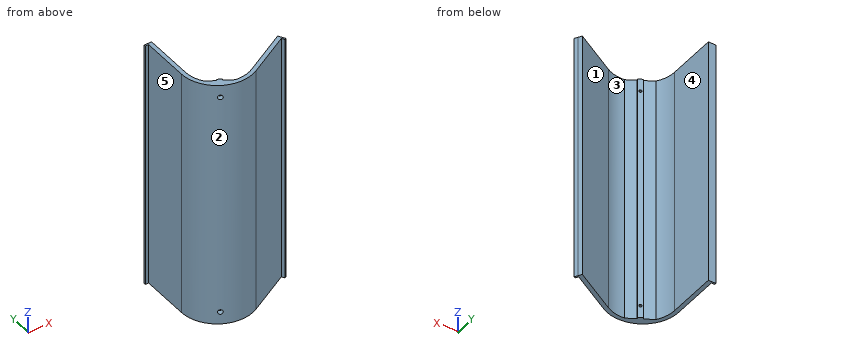
from build123d import *

# Parameters (mm, degrees)
BOSS_EXTRUDE1_DEPTH = 300
SKETCH3_R           = 1.6
CUT_EXTRUDE1_DEPTH  = 27.070508076
CUT_EXTRUDE2_START  = -2
SKETCH4_R           = 2.875
CUT_EXTRUDE2_DEPTH  = 25.070508162
SKETCH5_W           = 6
SKETCH5_H           = 300
SKETCH5_R           = 1.6
BOSS_EXTRUDE2_DEPTH = 2


with BuildPart() as part:
    # Sketch2 → Boss-Extrude1 (new body)
    with BuildSketch(Plane.XY):
        with BuildLine():
            Line((-10, 0), (-10, 57.592991829))
            Line((-10, 57.592991829), (-14, 57.592991829))
            Line((-14, 57.592991829), (-14, 59.592991829))
            Line((-14, 59.592991829), (-10, 59.592991829))
            Line((-10, 59.592991829), (-5, 59.592991829))
            Line((-5, 59.592991829), (-5, 0))
            ThreePointArc((-5, 0), (-3.13691529, -11.76748288), (2.270101024, -22.383928263))
            Line((2.270101024, -22.383928263), (29.120915128, -37.886253013))
            ThreePointArc((29.120915128, -37.886253013), (41.018534684, -37.260643809), (52.141016151, -32.990381057))
            Line((52.141016151, -32.990381057), (103.750060963, -3.193885142))
            Line((103.750060963, -3.193885142), (106.250060963, -7.524012161))
            Line((106.250060963, -7.524012161), (108.250060963, -10.988113776))
            Line((108.250060963, -10.988113776), (106.518010155, -11.988113776))
            Line((106.518010155, -11.988113776), (104.518010155, -8.524012161))
            Line((104.518010155, -8.524012161), (54.641016151, -37.320508076))
            ThreePointArc((54.641016151, -37.320508076), (11.547005384, -37.320508076), (-10, 0))
        make_face()
    extrude(amount=BOSS_EXTRUDE1_DEPTH)

    # Sketch3 → Cut-Extrude1 (cut, through all)
    with BuildSketch(Plane(origin=(-9.125, -15.804963619, 0), x_dir=(0.866025404, -0.5, 0), z_dir=(0.5, 0.866025404, 0))):
        with Locations((28.660254038, -15)):
            Circle(SKETCH3_R)
        with Locations((28.660254038, -285)):
            Circle(SKETCH3_R)
    extrude(amount=-CUT_EXTRUDE1_DEPTH, mode=Mode.SUBTRACT)

    # Sketch4 → Cut-Extrude2 (cut, through all)
    with BuildSketch(Plane(origin=(-9.125, -15.804963619, 0), x_dir=(0.866025404, -0.5, 0), z_dir=(0.5, 0.866025404, 0)).offset(CUT_EXTRUDE2_START)):
        with Locations((28.660254038, -15)):
            Circle(SKETCH4_R)
        with Locations((28.660254038, -285)):
            Circle(SKETCH4_R)
    extrude(amount=-CUT_EXTRUDE2_DEPTH, mode=Mode.SUBTRACT)

    # Sketch5 → Boss-Extrude2 (add)
    with BuildSketch(Plane(origin=(-9.125, -15.804963619, 0), x_dir=(0.866025404, -0.5, 0), z_dir=(0.5, 0.866025404, 0))):
        with Locations((28.660254038, -150)):
            Rectangle(SKETCH5_W, SKETCH5_H)
        with Locations((28.660254038, -15)):
            Circle(SKETCH5_R, mode=Mode.SUBTRACT)
        with Locations((28.660254038, -285)):
            Circle(SKETCH5_R, mode=Mode.SUBTRACT)
    extrude(amount=BOSS_EXTRUDE2_DEPTH)


solid = part.part
Verification items for the finished model (mm, model axes). Face numbers are marked on the shaded views. A direction names the side the tool comes from. Give positions to 0.01 mm unless a question says otherwise; leave off trailing zeros. Loops run counter-clockwise (first coordinate to the right, second up) from the corner with the lowest first, then second, coordinate; pieces in that order, holes last.
1. Material ranges on probe 1 along X at (y, z) = (23, 252.5); probe 2 along X at (y, z) = (-5.5, 170.5); probe 3 along X at (y, z) = (-18.5, 44.5), recorded low to high.
Derived:
probe 1: x = -10 to -5
probe 2: x = -9.65 to -4.6, 99.76 to 105.08
probe 3: x = -5.83 to -0.21, 77.24 to 87.24
2. Tool access check on the marked faces 1 and 2. Record the directions out of +Z, -Z, +X, -X, +Y, -Y that give a thin tool (end or side, any length) a straight path to the whole face; none if there is none.
Derived:
face 1: +Z, -Z, +Y
face 2: +Z, -Z, -Y
3. Cross-section at A-A on z = 61.5. Record the cut outline in (x, y).
Derived:
outline: (-14, 57.59) - (-10, 57.59) - (-10, 0) arc R43.09 ccw to (54.64, -37.32) - (104.52, -8.52) - (106.52, -11.99) - (108.25, -10.99) - (103.75, -3.19) - (52.14, -32.99) arc R38.09 cw to (29.12, -37.89) - (18.29, -31.64) - (19.29, -29.9) - (14.1, -26.9) - (13.1, -28.64) - (2.27, -22.38) arc R38.09 cw to (-5, 0) - (-5, 59.59) - (-14, 59.59) - close
4. Go/stop test with flat-tipped pins: P1, Ø3, axis at x = 50, z = 85.5, coming from the +Y side; P2, Ø8, axis at x = 3, z = 157, coming from the +Y side; P3, Ø12, axis at x = 24, z = 232.5, coming from the -Y side. Record where each tip stops, or that it passes through.
Derived:
P1: stops at y = -33.35
P2: stops at y = -16.99
P3: stops at y = -42.98
5. Cross-section at C-C on x = 25.5. Record the cut outline in (y, z).
Derived:
outline: (-42.42, 0) - (-35.8, 0) - (-35.8, 300) - (-42.42, 300) - close
6. Release check for a two-part mould opening along X. For the marked faces 3, 4 and 5 record: +X half, -X half, draft (parallel to the pull), parting line (faces both ways), or undercut.
Derived:
face 3: undercut
face 4: +X half
face 5: -X half
7. Cross-section at B-B on y = 25.5. Record the cut outline in (x, z), and give its area (3 significant figures).
Derived:
outline: (-10, 0) - (-5, 0) - (-5, 300) - (-10, 300) - close
area: 1,500 mm2
